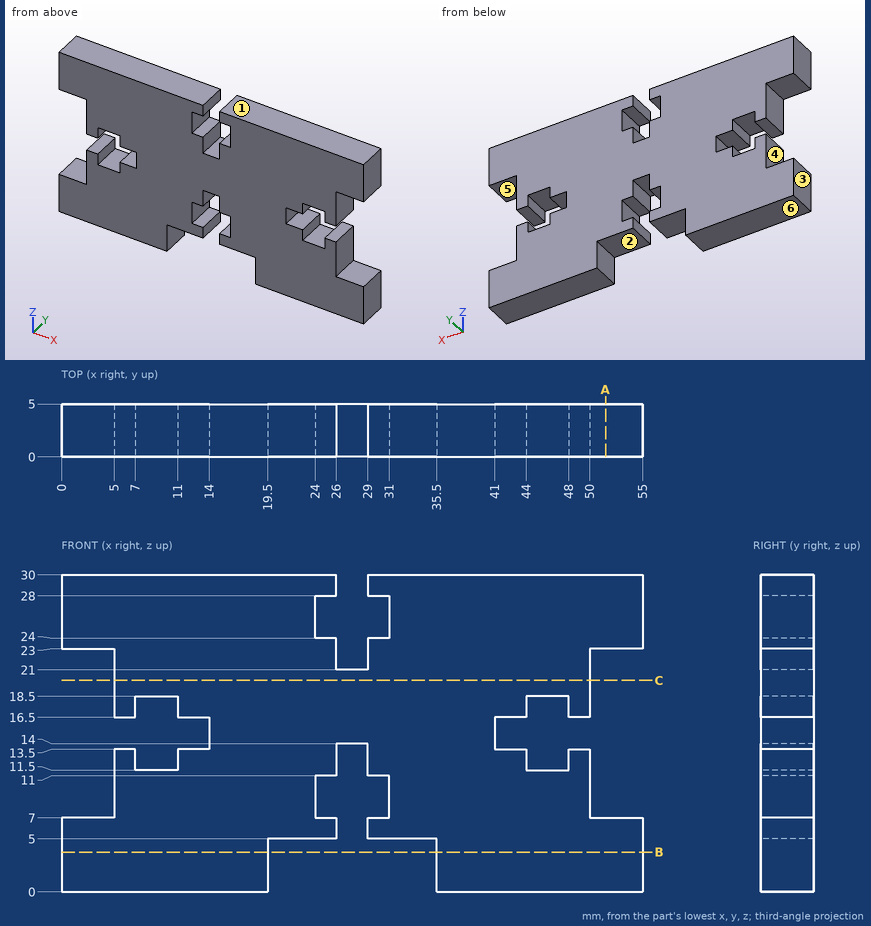
Input: dimensioned drawing with shaded views. Units: mm. Origin: part minimum x, y, z. A direction names the side the tool comes from. Give positions to 0.01 mm unless a question says otherwise; leave off trailing zeros. Loops run counter-clockwise (first coordinate to the right, second up) from the corner with the lowest first, then second, coordinate; pieces in that order, holes last. Notation, with made-up numbers: M 59.5,-11 L 66.5,-11 A17 ccw 66.5,-1 Z; hole C -14.5,28 d2. An arc over 180 degrees is marked long. Put each result on its own line as item: value. Start each with the question number.
1) Cut plane C-C (z = 20). Output: boundary loops of the cut face in (x, y).
2) Ray query, line 1 along Z through (x, y) = (30.5, 3.65); line 2 along X through (y, z) = (3.9, 17.5); line 3 along X through (y, z) = (2.55, 25.25). Return the intervals inside material, ascending.
3) Cut plane B-B (z = 3.75). Output: boundary loops of the cut face in (x, y).
4) Access query for the marked faces 4, 5 and 6. Directions: +Z, -Z, +X, -X, +Y, -Y. A direction counts if a zero-diameter tool reaches every point of the face in a straight line with its end or side. Return the directions, or none.
5) Pull-direction query (X, two-part tool) for the marked faces 1, 2 and 3; classes: pulls with the +X half, pulls with the -X half, needs draft (parallel to the pull), parting line crosses it, or undercut.
6) Cut plane A-A (x = 51.5). Output: boundary loops of the cut face in (y, z).
7) Contact query for flat-ended pins moving along their axis: pin 1 (1.5 mm diameter, centred on x = 31, y = 1.5, fed in from -Z); pin 2 (2 mm diameter, centred on y = 3, z = 16.5, fed in from -X); pin 3 (1.2 mm diameter, centred on x = 45, y = 3, fed in from -Z); pin 4 (1.5 mm diameter, centred on y = 2, z = 14.5, fed in from +X). Output: stop coordinate, or through.
Verdict:
1. outline: M 5,0 L 50,0 L 50,5 L 5,5 Z
2. line 1: 5 to 7, 11 to 24, 28 to 30
2. line 2: 5 to 7, 11 to 44, 48 to 50
2. line 3: 0 to 24, 31 to 55
3. outline: M 0,0 L 19.5,0 L 19.5,5 L 0,5 Z; M 35.5,0 L 55,0 L 55,5 L 35.5,5 Z
4. face 4: -X, +Y, -Y
4. face 5: +X, +Y, -Y
4. face 6: -Z, +X, -X, +Y, -Y
5. face 1: needs draft
5. face 2: undercut
5. face 3: pulls with the -X half
6. outline: M 0,0 L 5,0 L 5,7 L 0,7 Z; M 0,23 L 5,23 L 5,30 L 0,30 Z
7. pin 1: z = 5
7. pin 2: x = 5
7. pin 3: z = 0
7. pin 4: x = 41
